CAD build for the part. Positions are in the model's coordinates, mm. Round coordinates to 2 decimals unless told otherwise and drop trailing zeros. Loops run counter-clockwise (first coordinate to the right, second up) from the corner with the lowest first, then second, coordinate; pieces in that order, holes last.
```python
from build123d import *

# Parameters (mm, degrees)
CROQUIS1_W              = 120.365138791
CROQUIS1_H              = 200
SALIENTE_EXTRUIR1_DEPTH = 12
CORTAR_EXTRUIR1_REACH   = 126.056
CROQUIS2_R              = 3


with BuildPart() as part:
    # Croquis1 → Saliente-Extruir1 (new body)
    with BuildSketch(Plane.XY):
        with Locations((-1.236709328, 7.114481003)):
            Rectangle(CROQUIS1_W, CROQUIS1_H)
    extrude(amount=SALIENTE_EXTRUIR1_DEPTH)

    # Croquis2 → Cortar-Extruir1 (cut, up to next)
    with BuildSketch(Plane.XY.offset(12), mode=Mode.PRIVATE) as cortar_extruir1_sk1:
        with Locations((-12, 27.114481003)):
            Circle(CROQUIS2_R)
    cortar_extruir1_tool1 = extrude(cortar_extruir1_sk1.sketch, amount=-CORTAR_EXTRUIR1_REACH, mode=Mode.PRIVATE) & part.part
    # Croquis2 → Cortar-Extruir1 (cut, up to next)
    with BuildSketch(Plane.XY.offset(12), mode=Mode.PRIVATE) as cortar_extruir1_sk2:
        with Locations((12, 27.114481003)):
            Circle(CROQUIS2_R)
    cortar_extruir1_tool2 = extrude(cortar_extruir1_sk2.sketch, amount=-CORTAR_EXTRUIR1_REACH, mode=Mode.PRIVATE) & part.part
    # Croquis2 → Cortar-Extruir1 (cut, up to next)
    with BuildSketch(Plane.XY.offset(12), mode=Mode.PRIVATE) as cortar_extruir1_sk3:
        with Locations((-12, -12.885518997)):
            Circle(CROQUIS2_R)
    cortar_extruir1_tool3 = extrude(cortar_extruir1_sk3.sketch, amount=-CORTAR_EXTRUIR1_REACH, mode=Mode.PRIVATE) & part.part
    # Croquis2 → Cortar-Extruir1 (cut, up to next)
    with BuildSketch(Plane.XY.offset(12), mode=Mode.PRIVATE) as cortar_extruir1_sk4:
        with Locations((12, -12.885518997)):
            Circle(CROQUIS2_R)
    cortar_extruir1_tool4 = extrude(cortar_extruir1_sk4.sketch, amount=-CORTAR_EXTRUIR1_REACH, mode=Mode.PRIVATE) & part.part
    add(cortar_extruir1_tool1.solids().sort_by_distance((-12, 27.114481, 12))[0], mode=Mode.SUBTRACT)
    add(cortar_extruir1_tool2.solids().sort_by_distance((12, 27.114481, 12))[0], mode=Mode.SUBTRACT)
    add(cortar_extruir1_tool3.solids().sort_by_distance((-12, -12.885519, 12))[0], mode=Mode.SUBTRACT)
    add(cortar_extruir1_tool4.solids().sort_by_distance((12, -12.885519, 12))[0], mode=Mode.SUBTRACT)


solid = part.part
```
Item 1: Cut at A-A, the plane x = -12. Give the cut face in (y, z), plus the area to 3 significant figures.
Answers follow:
outline: (-92.89, 0) - (-15.89, 0) - (-15.89, 12) - (-92.89, 12) - close; (-9.89, 0) - (24.11, 0) - (24.11, 12) - (-9.89, 12) - close; (30.11, 0) - (107.11, 0) - (107.11, 12) - (30.11, 12) - close
area: 2,260 mm2
Item 2: Flat gauge pin, fed straight in: P1, Ø8, axis at x = 12, y = 27.11, coming from the +Z side. Where does the tip first touch, or does it go through?
Answers follow:
P1: stops at z = 12
Item 3: Probe line 1 (Y direction, x = 12, z = 7); line 2 (Y direction, x = -11, z = 9.5). List the from-to ranges inside material, lowest first.
Answers follow:
line 1: y = -92.89 to -15.89, -9.89 to 24.11, 30.11 to 107.11
line 2: y = -92.89 to -15.71, -10.06 to 24.29, 29.94 to 107.11
Item 4: Two-plate mould, pull along Y, no slides. Class faces 1 (the cylindrical face through (9.62, -14.71, 6.08)), 2 (the flat face through (-2, 107.114, 6)), 3 (the flat face through (-2, -92.886, 6)), 4 (the flat face through (-2, 9, 0)): released by +Y, released by -Y, zero draft, split by the parting line, or undercut.
Answers follow:
face 1: undercut
face 2: released by +Y
face 3: released by -Y
face 4: zero draft
